Verification items for the finished model (mm, model axes). A direction names the side the tool comes from. Round coordinates to 2 decimals unless told otherwise and drop trailing zeros. Loops run counter-clockwise (first coordinate to the right, second up) from the corner with the lowest first, then second, coordinate; pieces in that order, holes last. Notation, with made-up numbers: (-1.75, -32.75) -> (18.25, -32.75) arc R18 ccw to (18.25, -9.75) -> close; hole circle Ø6 at (61, -6.75). An arc over 180 degrees is marked (long way). Write item = value, one per line. Start each with the question number.
```python
from build123d import *

# Parameters (mm, degrees)
SKETCH1_W           = 15.89
SKETCH1_H           = 7.86
BOSS_EXTRUDE1_DEPTH = 3.15
SKETCH2_W           = 1.71
SKETCH2_H           = 1.04
CUT_EXTRUDE1_DEPTH  = 17.669118153
SKETCH3_W           = 12.79
SKETCH3_H           = 1.71
CUT_EXTRUDE2_DEPTH  = 10.111532528
SKETCH4_W           = 4.93
SKETCH4_H           = 2.11
CUT_EXTRUDE3_DEPTH  = 1.6


with BuildPart() as part:
    # Sketch1 → Boss-Extrude1 (new body)
    with BuildSketch(Plane(origin=(0, 0, 0), x_dir=(1, 0, 0), z_dir=(0, 1, 0))):
        Rectangle(SKETCH1_W, SKETCH1_H)
    extrude(amount=-BOSS_EXTRUDE1_DEPTH)

    # Sketch2 → Cut-Extrude1 (cut, through all)
    with BuildSketch(Plane(origin=(7.945, 0, 0), x_dir=(0, 0, -1), z_dir=(1, 0, 0))):
        with Locations((1.595, -0.52)):
            Rectangle(SKETCH2_W, SKETCH2_H)
        with Locations((-1.595, -0.52)):
            Rectangle(SKETCH2_W, SKETCH2_H)
    extrude(amount=-CUT_EXTRUDE1_DEPTH, mode=Mode.SUBTRACT)

    # Sketch3 → Cut-Extrude2 (cut, through all)
    with BuildSketch(Plane(origin=(0, -1.04, 0), x_dir=(1, 0, 0), z_dir=(0, 1, 0))):
        with Locations((0, 1.595)):
            Rectangle(SKETCH3_W, SKETCH3_H)
        with Locations((0, -1.595)):
            Rectangle(SKETCH3_W, SKETCH3_H)
    extrude(amount=-CUT_EXTRUDE2_DEPTH, mode=Mode.SUBTRACT)

    # Sketch4 → Cut-Extrude3 (cut)
    with BuildSketch(Plane.XY.offset(0.74)):
        with Locations((-3.93, -2.095)):
            Rectangle(SKETCH4_W, SKETCH4_H)
        with Locations((3.93, -2.095)):
            Rectangle(SKETCH4_W, SKETCH4_H)
    extrude(amount=-CUT_EXTRUDE3_DEPTH, mode=Mode.SUBTRACT)


solid = part.part
```
(1) Section check C-C on y = -0.15. Enter the section's corners in (x, z) (3 decimals).
(2) Section check D-D on z = 2. Enter the section's corners in (x, y) (3 decimals).
(3) Draft check along Z on faces 4 (the flat face through (0, -3.15, 0)), 5 (the flat face through (-7, -1.04, 2)), 6 (the flat face through (0, -2, 3.93)). Enter one of: +Z half, -Z half, draft (parallel to the pull), parting line (faces both ways), or undercut.
(4) Access from +Z, -Z, +X, -X, +Y, -Y to the whole of each face (thin tool, end or side, straight path). Record for faces 1 (the flat face through (0, -1, 0.74)), 2 (the flat face through (1.465, -2, 0)), 3 (the flat face through (7, -1.04, -2)).
(5) Section check A-A on x = -4.5. Enter the section's corners in (y, z), then the cut area to 3 significant figures.
(6) Depth check by flat-ended pin: pin 1 Ø0.7 at (x, z) = (4, 0) entering from -Y; pin 2 Ø0.5 at (x, z) = (-7, 2) entering from +Y. Enter the tip coordinate at first touch or a pass-through.
(7) Section check B-B on y = -1.6. Enter the section's corners in (x, z) (3 decimals), then the cut area to 3 significant figures.
(8) Scan lines: line 1 (X direction, y = -2.3, z = -0.25) (3 decimals); line 2 (Z direction, x = -2.25, y = -0.3); line 3 (Z direction, x = -1.75, y = -2.4). Record each from-to range of solid material in increasing order. Write a range as [from, to].
Computed values:
q1.outline = (-7.945, -3.93) -> (7.945, -3.93) -> (7.945, -2.45) -> (-7.945, -2.45) -> close; (-7.945, -0.74) -> (7.945, -0.74) -> (7.945, 0.74) -> (-7.945, 0.74) -> close; (-7.945, 2.45) -> (7.945, 2.45) -> (7.945, 3.93) -> (-7.945, 3.93) -> close
q2.outline = (-7.945, -3.15) -> (-6.395, -3.15) -> (-6.395, -1.04) -> (-7.945, -1.04) -> close; (6.395, -3.15) -> (7.945, -3.15) -> (7.945, -1.04) -> (6.395, -1.04) -> close
q3.face_4 = draft
q3.face_5 = undercut
q3.face_6 = +Z half
q4.face_1 = +Y
q4.face_2 = -Y
q4.face_3 = +X, -X, +Y
q5.outline = (-3.15, -3.93) -> (0, -3.93) -> (0, -2.45) -> (-3.15, -2.45) -> close; (-3.15, 2.45) -> (0, 2.45) -> (0, 3.93) -> (-3.15, 3.93) -> close; (-1.04, -0.74) -> (0, -0.74) -> (0, 0.74) -> (-1.04, 0.74) -> close
q5.area = 10.9 mm²
q6.pin_1 = -1.04
q6.pin_2 = -1.04
q7.outline = (-7.945, -3.93) -> (7.945, -3.93) -> (7.945, 3.93) -> (-7.945, 3.93) -> close; (-1.465, -0.74) -> (1.465, -0.74) -> (1.465, 0.74) -> (-1.465, 0.74) -> close; hole (-6.395, -2.45) -> (6.395, -2.45) -> (6.395, 2.45) -> (-6.395, 2.45) -> close
q7.area = 66.6 mm²
q8.line_1 = [-7.945, -6.395], [-1.465, 1.465], [6.395, 7.945]
q8.line_2 = [-3.93, -2.45], [-0.74, 0.74], [2.45, 3.93]
q8.line_3 = [-3.93, -2.45], [2.45, 3.93]
